Check sheet for the drawn part. Datum: minimum x, y, z corner. Units: mm. A direction names the side the tool comes from. Round coordinates to 2 decimals unless told otherwise and drop trailing zeros. Write each loop counter-clockwise with the first axis right and the second up, starting at its lowest first coordinate (ties: lowest second). Pieces come first, ordered by that corner, then holes.
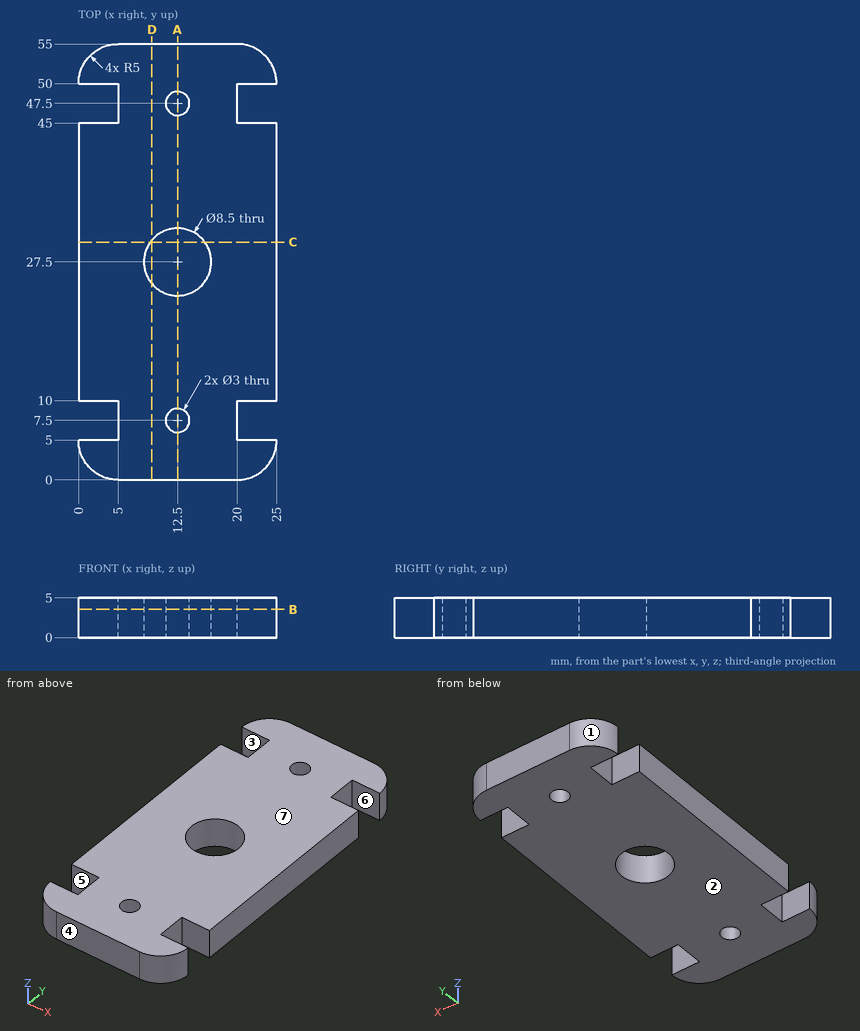
1. Sectioned sample at A-A, the plane x = 12.5. Enter the section's corners in (y, z).
2. Release check for a two-part mould opening along Y. For the marked faces 1, 2, 3 and 4 record: released by +Y, released by -Y, zero draft, split by the parting line, or undercut.
3. Sectioned sample at B-B, the plane z = 3.55. Give the number of separate pieces and of enclosed holes in the cut face, plus the area to 3 significant figures.
4. Set-up check for the marked faces 5, 6 and 7: record each of +Z, -Z, +X, -X, +Y, -Y from which the full face is reachable in a straight line by a thin tool's end or side.
5. Sectioned sample at D-D, the plane x = 9.25. Enter the section's corners in (y, z).
6. Go/stop test with flat-tipped pins: pin 1 (1.5 mm diameter, centred on x = 23, z = 1.5, fed in from -Y) (3 decimals); pin 2 (2.5 mm diameter, centred on x = 3, z = 3.5, fed in from +Y); pin 3 (4 mm diameter, centred on x = 12.5, y = 47.5, fed in from -Z); pin 4 (1.5 mm diameter, centred on x = 22.5, z = 2.5, fed in from +Y). Record where each tip stops, or that it passes through.
7. Sectioned sample at C-C, the plane y = 30. Enter the section's corners in (x, z), plus the area to 3 significant figures.
8. Scan lines: line 1 along Y through (x, z) = (12.5, 1.8); line 2 along Y through (x, z) = (2.5, 1); line 3 along X through (y, z) = (46.5, 3.75). Record each from-to range of solid material in increasing order.
Computed values:
1. outline: (0, 0) - (6, 0) - (6, 5) - (0, 5) - close; (9, 0) - (23.25, 0) - (23.25, 5) - (9, 5) - close; (31.75, 0) - (46, 0) - (46, 5) - (31.75, 5) - close; (49, 0) - (55, 0) - (55, 5) - (49, 5) - close
2. face 1: released by +Y
2. face 2: zero draft
2. face 3: undercut
2. face 4: released by -Y
3. separate pieces: 1
3. enclosed holes: 3
3. area: 1,180 mm2
4. face 5: +Z, -Z, -X
4. face 6: +Z, -Z, +X
4. face 7: +Z, +X, -X, +Y, -Y
5. outline: (0, 0) - (24.76, 0) - (24.76, 5) - (0, 5) - close; (30.24, 0) - (55, 0) - (55, 5) - (30.24, 5) - close
6. pin 1: stops at y = 0.535
6. pin 2: stops at y = 54.94
6. pin 3: stops at z = 0
6. pin 4: stops at y = 54.68
7. outline: (0, 0) - (9.06, 0) - (9.06, 5) - (0, 5) - close; (15.94, 0) - (25, 0) - (25, 5) - (15.94, 5) - close
7. area: 90.6 mm2
8. line 1: y = 0 to 6, 9 to 23.25, 31.75 to 46, 49 to 55
8. line 2: y = 0.67 to 5, 10 to 45, 50 to 54.33
8. line 3: x = 5 to 11.38, 13.62 to 20
